Verification items for the finished model (mm, model axes). Face numbers are marked on the shaded views. A direction names the side the tool comes from. Give positions to 0.01 mm unless a question says otherwise; leave off trailing zeros. Order: outer loops, then holes, each group sorted by start corner. A loop starts at its lowest first (then second) coordinate and runs counter-clockwise, first axis right, second up.
from build123d import *

# Parameters (mm, degrees)
F1_DEPTH = 101.6
F3_DEPTH = 40.894
F5_DEPTH = 25.401


with BuildPart() as f1:
    # F0 (on Front) → F1 (new body, symmetric)
    with BuildSketch(Plane.XZ):
        Polygon((101.6, 0), (0, 0), (0, -25.4), (127, -25.4), (177.8, 25.4), (228.6, -25.4), (254, 0), (127, 127), (101.6, 101.6), (152.4, 50.8), align=None)
    extrude(amount=F1_DEPTH, both=True)

    # F2 (on face) → F3 (cut)
    with BuildSketch(Plane(origin=(127, 0, 127), x_dir=(0, 1, 0), z_dir=(0.707107, 0, 0.707107))):
        with BuildLine():
            ThreePointArc((-50.8, -19.05), (-37.329616, -24.629616), (-31.75, -38.1))
            ThreePointArc((-31.75, -38.1), (-37.329616, -51.570384), (-50.8, -57.15))
            Line((-50.8, -57.15), (50.8, -57.15))
            ThreePointArc((50.8, -57.15), (31.75, -38.1), (50.8, -19.05))
            Line((50.8, -19.05), (-50.8, -19.05))
        make_face()
        with BuildLine():
            ThreePointArc((-50.8, -57.15), (-37.329616, -51.570384), (-31.75, -38.1))
            ThreePointArc((-31.75, -38.1), (-37.329616, -24.629616), (-50.8, -19.05))
            ThreePointArc((-50.8, -19.05), (-69.85, -38.1), (-50.8, -57.15))
        make_face()
        with BuildLine():
            ThreePointArc((69.85, -38.1), (64.270384, -24.629616), (50.8, -19.05))
            ThreePointArc((50.8, -19.05), (31.75, -38.1), (50.8, -57.15))
            ThreePointArc((50.8, -57.15), (64.270384, -51.570384), (69.85, -38.1))
        make_face()
        with BuildLine():
            ThreePointArc((69.85, -141.505122), (64.270384, -128.034738), (50.8, -122.455122))
            ThreePointArc((50.8, -122.455122), (31.75, -141.505122), (50.8, -160.555122))
            ThreePointArc((50.8, -160.555122), (64.270384, -154.975507), (69.85, -141.505122))
        make_face()
        with BuildLine():
            ThreePointArc((-50.8, -122.455122), (-37.329616, -128.034738), (-31.75, -141.505122))
            ThreePointArc((-31.75, -141.505122), (-37.329616, -154.975507), (-50.8, -160.555122))
            Line((-50.8, -160.555122), (50.8, -160.555122))
            ThreePointArc((50.8, -160.555122), (31.75, -141.505122), (50.8, -122.455122))
            Line((50.8, -122.455122), (-50.8, -122.455122))
        make_face()
        with BuildLine():
            ThreePointArc((-50.8, -160.555122), (-37.329616, -154.975507), (-31.75, -141.505122))
            ThreePointArc((-31.75, -141.505122), (-37.329616, -128.034738), (-50.8, -122.455122))
            ThreePointArc((-50.8, -122.455122), (-69.85, -141.505122), (-50.8, -160.555122))
        make_face()
    extrude(amount=-F3_DEPTH, mode=Mode.SUBTRACT)

    # F4 (on face) → F5 (cut, through all)
    with BuildSketch(Plane.XY):
        with BuildLine():
            Line((0, -12.7), (50.8, -12.7))
            ThreePointArc((50.8, -12.7), (63.5, 0), (50.8, 12.7))
            Line((50.8, 12.7), (0, 12.7))
            Line((0, 12.7), (0, 0))
            Line((0, 0), (0, -12.7))
        make_face()
    extrude(amount=-F5_DEPTH, mode=Mode.SUBTRACT)


solid = f1.part
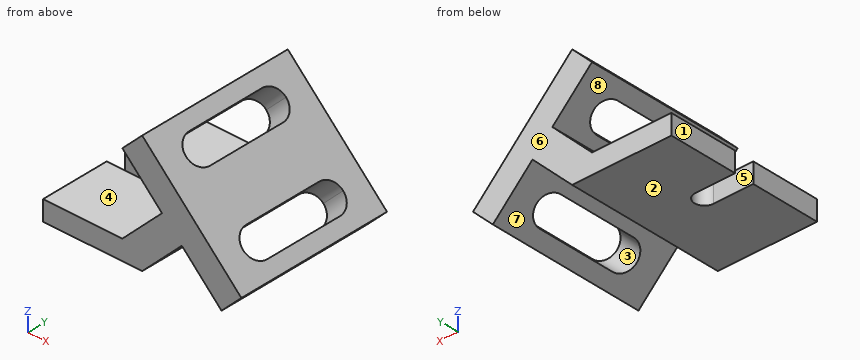
(1) Go/stop test with flat-tipped pins: pin 1 (6 mm diameter, centred on y = -68.5, z = 81, fed in from -X); pin 2 (6 mm diameter, centred on y = -26.5, z = 46.5, fed in from -X); pin 3 (5 mm diameter, centred on y = 36.5, z = 91.5, fed in from +X). Record where each tip stops, or that it passes through.
Solved:
pin 1: stops at x = 119.2
pin 2: stops at x = 145.1
pin 3: stops at x = 120.94
(2) Section check A-A, the plane y = 25.5. Enter the section's corners in (x, z).
Solved:
outline: (0, -25.4) - (127, -25.4) - (177.8, 25.4) - (188.19, 15.01) - (213.59, 40.41) - (167.41, 86.59) - (142.01, 61.19) - (152.4, 50.8) - (101.6, 0) - (0, 0) - close; (101.6, 101.6) - (115.07, 88.13) - (140.47, 113.53) - (127, 127) - close; (215.13, -11.93) - (228.6, -25.4) - (254, 0) - (240.53, 13.47) - close
(3) Section check B-B, the plane x = 26. Enter the section's corners in (y, z), then the cut area to 3 significant figures.
Solved:
outline: (-101.6, -25.4) - (-12.7, -25.4) - (-12.7, 0) - (-101.6, 0) - close; (12.7, -25.4) - (101.6, -25.4) - (101.6, 0) - (12.7, 0) - close
area: 4,520 mm2
(4) Section check C-C, the plane y = 0. Enter the section's corners in (x, z).
Solved:
outline: (63.5, -25.4) - (127, -25.4) - (177.8, 25.4) - (188.19, 15.01) - (213.59, 40.41) - (167.41, 86.59) - (142.01, 61.19) - (152.4, 50.8) - (101.6, 0) - (63.5, 0) - close; (101.6, 101.6) - (115.07, 88.13) - (140.47, 113.53) - (127, 127) - close; (215.13, -11.93) - (228.6, -25.4) - (254, 0) - (240.53, 13.47) - close
(5) Release check for a two-part mould opening along Z. For the marked faces 1, 2 and 3 record: pulls with the +Z half, pulls with the -Z half, needs draft (parallel to the pull), parting line crosses it, or undercut.
Solved:
face 1: needs draft
face 2: pulls with the -Z half
face 3: undercut
(6) Scan lines: line 1 (Y direction, x = 208, z = 7.5); line 2 (Z direction, x = 53, y = -78); line 3 (Y direction, x = 18, z = -19). Record each from-to range of solid material in increasing order.
Solved:
line 1: y = -101.6 to -69.85, 69.85 to 101.6
line 2: z = -25.4 to 0
line 3: y = -101.6 to -12.7, 12.7 to 101.6
(7) Set-up check for the marked faces 4, 5, 6, 7 and 8: record each of +Z, -Z, +X, -X, +Y, -Y from which the full face is reachable in a straight line by a thin tool's end or side.
Solved:
face 4: +Z, -X, +Y, -Y
face 5: +Z, -Z, -X
face 6: +Z, -Z, +X, -X, +Y
face 7: -Z, +Y, -Y
face 8: -X, +Y, -Y
